Part model, mm, in its own coordinate system. A direction names the side the tool comes from. Give positions to 0.01 mm unless a question says otherwise; leave off trailing zeros. Write each loop counter-clockwise with the first axis right and the second up, starting at its lowest first coordinate (ties: lowest second). Pieces come first, ordered by that corner, then holes. Notation, with made-up numbers: M -15.75,-5 L -4.75,-5 A26 cw -4.75,34 Z; hole C 15.5,-34.5 d3. An arc over 180 degrees is marked long. Use a Markdown table: item, result.
```python
from build123d import *

# Parameters (mm, degrees)
SKETCH_1_R          = 10
EXTRUDE_1_DEPTH     = 0.2
EXTRUDE_2_DEPTH     = 6
SKETCH_3_R          = 4
EXTRUDE_3_DEPTH     = 1.6
SKETCH_4_R          = 7
EXTRUDE_4_DEPTH     = 0.22
SKETCH_5_R          = 2
EXTRUDE_5_DEPTH     = 4
SKETCH_6_R          = 0.2
EXTRUDE_6_DEPTH     = 3
CUT_EXTRUDE_1_DEPTH = 1.5


with BuildPart() as part:
    # 草图1 → 凸台-拉伸1 (new body)
    with BuildSketch(Plane(origin=(0, 0, 0), x_dir=(1, 0, 0), z_dir=(0, 1, 0))):
        with Locations(Location((0, 0, 0), (0, 0, 270))):
            Circle(SKETCH_1_R)
    extrude(amount=EXTRUDE_1_DEPTH)

    # 草图2 → 凸台-拉伸2 (add)
    with BuildSketch(Plane(origin=(0, 0.2, 0), x_dir=(1, 0, 0), z_dir=(0, 1, 0))):
        Polygon((-0.8, 3), (0.8, 3), (0.8, 0.8), (3, 0.8), (3, -0.8), (0.8, -0.8), (0.8, -3), (-0.8, -3), (-0.8, -0.8), (-3, -0.8), (-3, 0.8), (-0.8, 0.8), align=None)
    extrude(amount=EXTRUDE_2_DEPTH)

    # 草图3 → 凸台-拉伸3 (add)
    with BuildSketch(Plane(origin=(0, 6.2, 0), x_dir=(1, 0, 0), z_dir=(0, 1, 0))):
        with Locations(Location((0, 0, 0), (0, 0, 270))):
            Circle(SKETCH_3_R)
    extrude(amount=EXTRUDE_3_DEPTH)

    # 草图4 → 凸台-拉伸4 (add)
    with BuildSketch(Plane(origin=(0, 0, 0), x_dir=(-1, 0, 0), z_dir=(0, -1, 0))):
        with Locations(Location((0, 0, 0), (0, 0, 90))):
            Circle(SKETCH_4_R)
    extrude(amount=EXTRUDE_4_DEPTH)

    # 草图5 → 凸台-拉伸5 (add)
    with BuildSketch(Plane(origin=(0, 7.8, 0), x_dir=(1, 0, 0), z_dir=(0, 1, 0))):
        with Locations(Location((0, 0, 0), (0, 0, 270))):
            Circle(SKETCH_5_R)
    extrude(amount=EXTRUDE_5_DEPTH)

    # 草图6 → 凸台-拉伸6 (add)
    with BuildSketch(Plane(origin=(0, 11.8, 0), x_dir=(1, 0, 0), z_dir=(0, 1, 0))):
        with Locations(Location((0, 0, 0), (0, 0, 270))):
            Circle(SKETCH_6_R)
    extrude(amount=EXTRUDE_6_DEPTH)

    # 草图7 → 切除-拉伸1 (cut, symmetric)
    with BuildSketch(Plane(origin=(0, 0, 0), x_dir=(0, 0, -1), z_dir=(1, 0, 0))):
        Polygon((0.2, 14.8), (-0.2, 14.8), (-0.2, 13.740589274), align=None)
    extrude(amount=CUT_EXTRUDE_1_DEPTH, both=True, mode=Mode.SUBTRACT)


solid = part.part
```
1. Cut at D-D, the plane z = 4.75. Give the cut face in (x, y), then the cut area to 3 significant figures.
Findings below:
| item | result |
|---|---|
| outline | M -8.8,0 L -5.14,0 L -5.14,-0.22 L 5.14,-0.22 L 5.14,0 L 8.8,0 L 8.8,0.2 L -8.8,0.2 Z |
| area | 5.78 mm2 |
2. Drop flat-ended pins along their axis: P1, Ø1.5, axis at x = -7, z = -5, coming from the -Y side; P2, Ø1.8, axis at x = -1.5, y = 4, coming from the +Z side; P3, Ø1.5, axis at x = -5.5, y = 9, coming from the -Z side; P4, Ø0.7, axis at y = 4, z = -2, coming from the +X side. Give the stop position or say it passes through.
Findings below:
| item | result |
|---|---|
| P1 | y = 0 |
| P2 | z = 3 |
| P3 | through |
| P4 | x = 0.8 |
3. Drill centre lines: L1, parallel to Y at x = 0, z = 3.5; L2, parallel to X at y = 1.5, z = 1.25; L3, parallel to Y at x = -1.75, z = -6.25. Where is each one in solid material? Low to high.
Findings below:
| item | result |
|---|---|
| L1 | -0.22 to 0.2, 6.2 to 7.8 |
| L2 | -0.8 to 0.8 |
| L3 | -0.22 to 0.2 |
4. Cut at B-B, the plane z = -3.5. Give the cut face in (x, y), then the cut area to 3 significant figures.
Findings below:
| item | result |
|---|---|
| outline | M -9.37,0 L -6.06,0 L -6.06,-0.22 L 6.06,-0.22 L 6.06,0 L 9.37,0 L 9.37,0.2 L -9.37,0.2 Z; M -1.94,6.2 L 1.94,6.2 L 1.94,7.8 L -1.94,7.8 Z |
| area | 12.6 mm2 |
5. Cut at C-C, the plane y = 2.75. Give the cut face in (x, z), then the cut area to 3 significant figures.
Findings below:
| item | result |
|---|---|
| outline | M -3,-0.8 L -0.8,-0.8 L -0.8,-3 L 0.8,-3 L 0.8,-0.8 L 3,-0.8 L 3,0.8 L 0.8,0.8 L 0.8,3 L -0.8,3 L -0.8,0.8 L -3,0.8 Z |
| area | 16.6 mm2 |
6. Tool access for faces 1 (the flat face through (0, 3, 3)), 2 (the flat face through (0, 3, -3)), 3 (the cylindrical face through (-2, 10, 0)): list every direction of +Z, -Z, +X, -X, +Y, -Y with a clear straight run to the whole face (end or side of a thin tool).
Findings below:
| item | result |
|---|---|
| face 1 | +Z, +X, -X |
| face 2 | -Z, +X, -X |
| face 3 | +Y |
7. Two-plate mould, pull along Y, no slides. Class faces 4 (the cylindrical face through (-3.905, 6.989, -0.867)), 5 (the flat face through (7, 0, 2)), 6 (the flat face through (-1, 6.2, 1)): released by +Y, released by -Y, zero draft, split by the parting line, or undercut.
Findings below:
| item | result |
|---|---|
| face 4 | zero draft |
| face 5 | released by -Y |
| face 6 | undercut |
8. Cut at A-A, the plane x = -3.5. Give the cut face in (y, z), then the cut area to 3 significant figures.
Findings below:
| item | result |
|---|---|
| outline | M -0.22,-6.06 L 0,-6.06 L 0,-9.37 L 0.2,-9.37 L 0.2,9.37 L 0,9.37 L 0,6.06 L -0.22,6.06 Z; M 6.2,-1.94 L 7.8,-1.94 L 7.8,1.94 L 6.2,1.94 Z |
| area | 12.6 mm2 |
